Design review of the part shown in the three views and the two pictorial views. Dimensions are in mm from the part's minimum x, y and z. Coordinates: 2 decimals unless noted, no trailing zeros. Loops run counter-clockwise (first coordinate to the right, second up) from the corner with the lowest first, then second, coordinate; pieces in that order, holes last.
Q1. Add section B-B on x = 15. Give the boundary of the cut face in (y, z), and give its area (3 significant figures).
Q2. Add section D-D on z = 20. Give the boundary of the cut face in (x, y), and give its area (3 significant figures).
Q3. For P1, Ø8, axis at y = 77.5, z = 46, coming from the +X side; P2, Ø3.5, axis at y = 29.45, z = 50, coming from the +X side; P3, Ø5, axis at y = 50, z = 50, coming from the -X side; P4, Ø2, axis at x = 62, y = 47, coming from the -Z side, all flat-tipped, find the tip position at first contact; note any pin that passes through.
Q4. Add section A-A on z = 50. Give the boundary of the cut face in (x, y) (3 decimals).
Q5. Wall thickness on probe 1 along Y at (x, z) = (3.8, 50) (3 decimals); probe 2 along X at (y, z) = (42, 18); probe 3 along Z at (x, y) = (18.5, 48): over which ranges is each line inside the solid? List them lowest first.
Q6. Add section C-C on y = 8. Give the boundary of the cut face in (x, z).
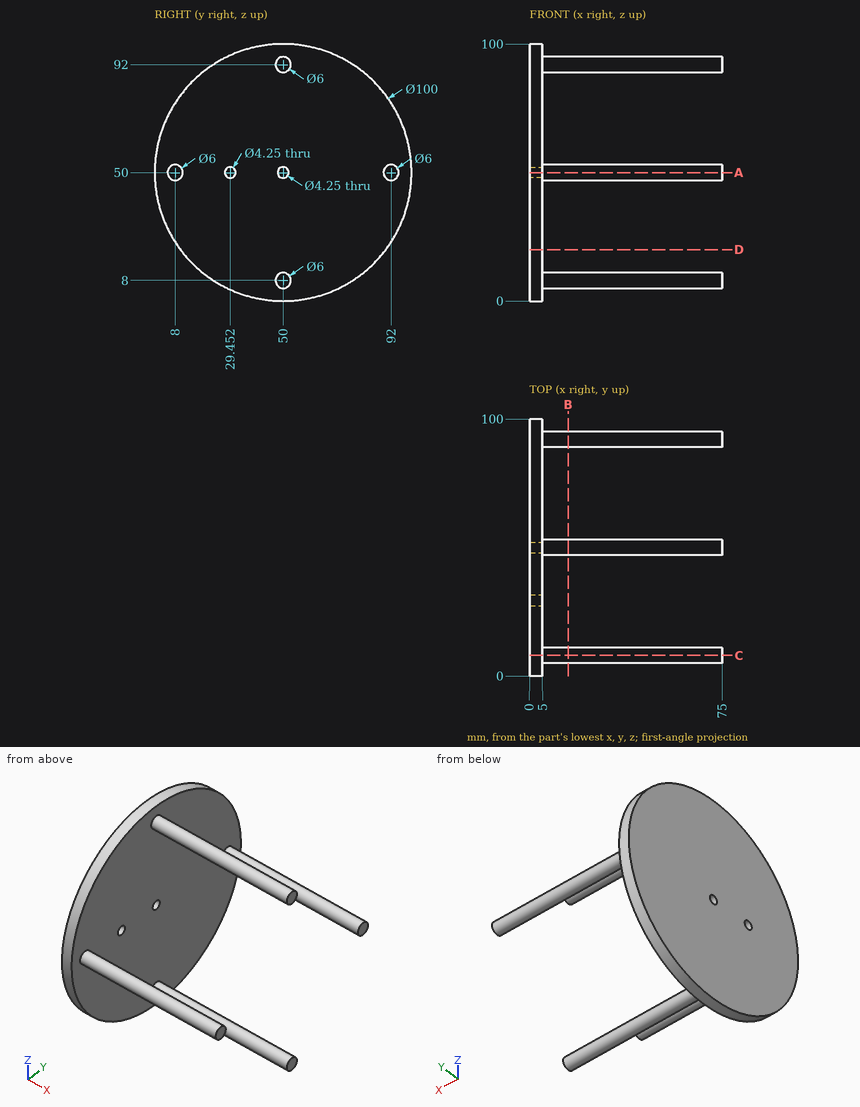
Entries:
1. outline: circle Ø6 at (8, 50); circle Ø6 at (50, 8); circle Ø6 at (50, 92); circle Ø6 at (92, 50)
1. area: 113 mm2
2. outline: (0, 10) - (5, 10) - (5, 90) - (0, 90) - close
2. area: 400 mm2
3. P1: stops at x = 5
3. P2: passes through
3. P3: stops at x = 0
3. P4: stops at z = 5.76
4. outline: (0, 0) - (5, 0) - (5, 5) - (75, 5) - (75, 11) - (5, 11) - (5, 27.327) - (0, 27.327) - close; (0, 31.577) - (5, 31.577) - (5, 47.875) - (0, 47.875) - close; (0, 52.125) - (5, 52.125) - (5, 89) - (75, 89) - (75, 95) - (5, 95) - (5, 100) - (0, 100) - close
5. probe 1: y = 0 to 27.327, 31.577 to 47.875, 52.125 to 100
5. probe 2: x = 0 to 5
5. probe 3: z = 5.76 to 10.24, 89.76 to 94.24
6. outline: (0, 22.87) - (5, 22.87) - (5, 47) - (75, 47) - (75, 53) - (5, 53) - (5, 77.13) - (0, 77.13) - close
